Geometry check sheet. Reference: the model listing, model coordinates, mm. A direction names the side the tool comes from. Round coordinates to 2 decimals unless told otherwise and drop trailing zeros. Order: outer loops, then holes, each group sorted by start corner. A loop starts at its lowest first (then second) coordinate and runs counter-clockwise, first axis right, second up.
(1) Cross-section at C-C on z = -2.5. Count the separate pieces of the cut face and the enclosed holes in it, and give its area (3 significant figures).
(2) Gauge pin test, flat ends, axial feed: P1, Ø3.5, axis at x = 0, z = -30.245, coming from the +Y side (3 decimals); P2, Ø3.5, axis at x = 0, y = 22.54, coming from the +Z side; P3, Ø4.5, axis at y = 12, z = -38.5, coming from the +X side. Record the tip position at first contact, or that the pin passes through.
(3) Draft check along Z on faces 6 (the face through (8.372, 1.61, -22.777)), 7 (the face through (0.564, 1.61, -14.112)), 8 (the face through (0, 0, -16)), 9 (the face through (1.3, 20.6, 0)). Enter one of: pulls with the +Z half, pulls with the -Z half, needs draft (parallel to the pull), parting line crosses it, or undercut.
(4) Thickness scan on L1, parallel to Y at x = 0, z = -39.2 (1 decimal); L2, parallel to Y at x = 0, z = -1.9 (1 decimal); L3, parallel to Z at x = 0, y = 1.3 (3 decimals). Record the ranges inside material, lowest first.
(5) Set-up check for faces 1 (the face through (6.35, 14, -38)), 2 (the face through (0.879, 20.852, -1.565)), 3 (the face through (-6.35, 13, -3)), 4 (the face through (-6.35, 13, -38)), 5 (the face through (3, 22, -3.175)): record each of +Z, -Z, +X, -X, +Y, -Y from which the full face is reachable in a straight line by a thin tool's end or side.
(6) Cross-section at B-B on x = -8. Enter the section's corners in (y, z) (3 decimals).
(7) Cross-section at A-A on y = 4.5. Enter the section's corners in (x, z) (3 decimals), and give its area (3 significant figures).
Autodesk Inventor part; units mm, degrees
ref_plane "YZ Plane" through (0, 0, 0) normal (1, 0, 0) x (0, 1, 0)
ref_plane "XZ Plane" through (0, 0, 0) normal (0, 1, 0) x (-1, 0, 0)
ref_plane "XY Plane" through (0, 0, 0) normal (0, 0, 1) x (1, 0, 0)
sketch "Sketch1" plane through (0, 0, 0) normal (0, 0, 1) x (1, 0, 0)
  line L0 (-6.35, 0) -> (-6.35, 3.175)
  line L1 (-6.35, 3.175) -> (-6.35, 34.29)
  line L2 (6.35, 34.29) -> (6.35, 3.175)
  line L3 (6.35, 3.175) -> (6.35, 0)
  line L4 (6.35, 0) -> (-6.35, 0)
  arc A0 (6.35, 34.29) -> (-6.35, 34.29) centre (0, 34.29) ccw
  point P0 (0, 0)
  point P1 (0, 0)
  dimension "d3" = 12.7
  dimension "d4" = 40.64
  dimension "d26" = 6.35
  dimension "d27" = 3.175
extrude "Extrusion1" add sketch "Sketch1" against normal blind 3.175
sketch "Sketch2" plane through (0, 0, -3.175) normal (0, 0, -1) x (-1, 0, 0)
  line L0 (-6.35, 34.29) -> (-6.35, 0)
  line L1 (6.35, 0) -> (-6.35, 0)
  line L2 (-6.35, 0) -> (-6.35, 3.175)
  line L3 (-6.35, 3.175) -> (6.35, 3.175)
  line L4 (6.35, 3.175) -> (6.35, 0)
  point P0 (0, 0)
  point P1 (-6.35, 3.175)
  dimension "d5" = 3.175
extrude "Extrusion2" add sketch "Sketch2" along normal blind 34.452
sketch "Sketch3" plane through (0, 0, -37.627) normal (0, 0, -1) x (-1, 0, 0)
  line L0 (-6.35, 0) -> (6.35, 0)
  line L1 (6.35, 0) -> (-6.35, 0)
  line L2 (6.35, 0) -> (6.35, 34.29)
  line L3 (-6.35, 3.175) -> (-6.35, 0)
  line L4 (-6.35, 0) -> (-6.35, 3.175)
  line L5 (-6.35, 3.175) -> (-6.35, 34.29)
  arc A0 (6.35, 34.29) -> (-6.35, 34.29) centre (0, 34.29) ccw
  point P0 (0, 0)
  dimension "d45" = 6.35
  dimension "d55" = 34.29
extrude "Extrusion7" add sketch "Sketch3" along normal blind 3.175
sketch "Sketch4" plane through (-6.35, 3.175, -3.175) normal (0, 1, 0) x (1, 0, 0)
  circle A0 centre (6.35, 17.226) radius 12.7
  line L0 (0, 0) -> (0, 34.452) construction
  line L1 (0, 0) -> (12.7, 34.452) construction
  point P0 (6.35, -3.175)
  point P1 (12.7, 34.452)
  dimension "d13" = 25.4
extrude "Extrusion4" add sketch "Sketch4" against normal up to surface (3.175 mm away)
sketch "Sketch6" plane through (0, 0, 0) normal (0, 0, 1) x (1, 0, 0)
  circle A0 centre (0, 34.29) radius 1.27
  circle A1 centre (0, 10.795) radius 1.27
  line L0 (0, 10.795) -> (0, 34.29) construction
  line L1 (6.35, 0) -> (-6.35, 0) construction
  line L2 (-1.27, 22.5425) -> (0, 22.5425) construction
  line L3 (-1.27, 10.795) -> (-1.27, 34.29) construction
  arc A2 (6.35, 34.29) -> (-6.35, 34.29) centre (0, 34.29) ccw
  line L4 (-6.35, 3.175) -> (-6.35, 34.29) construction
  line L5 (-6.35, 10.795) -> (6.35, 10.795) construction
  point P0 (0, 0)
  point P1 (0, 0)
  dimension "d18" = 2.54
  dimension "d19" = 23.495
extrude "Extrusion6" cut sketch "Sketch6" against normal blind 500
sketch "Sketch8" plane through (-6.35, 3.175, -3.175) normal (0, 1, 0) x (1, 0, 0)
  circle A0 centre (6.35, 17.226) radius 3.175
  arc A1 (0, 28.2245) -> (0, 6.2275) centre (6.35, 17.226) ccw
  point P0 (6.35, -3.175)
  dimension "d36" = 6.35
extrude "Extrusion9" cut sketch "Sketch8" against normal up to next
sketch "Sketch9" plane through (0, 0, 0) normal (0, 0, 1) x (1, 0, 0)
  circle A0 centre (0, 22.5425) radius 1.905
  circle A1 centre (0, 34.29) radius 1.27 construction
  circle A2 centre (0, 10.795) radius 1.27 construction
  line L0 (0, 34.29) -> (0, 10.795) construction
  point P0 (0, 0)
  point P1 (0, 22.5425)
  dimension "d39" = 3.81
extrude "Extrusion10" cut sketch "Sketch9" against normal up to next
sketch "Sketch10" plane through (-6.35, 3.175, -3.175) normal (0, 1, 0) x (1, 0, 0)
  circle A0 centre (6.35, 10.0521) radius 1.05
  circle A1 centre (-2.159, 18.5611) radius 1.05
  circle A2 centre (6.35, 27.07) radius 1.05
  circle A3 centre (14.859, 18.5611) radius 1.05
  point P0 (6.35, -3.175)
extrude "Extrusion11" cut sketch "Sketch10" against normal up to next
sketch "Sketch12" plane through (0, 0, -40.802) normal (0, 0, -1) x (-1, 0, 0)
  circle A0 centre (0, 22.5425) radius 1.651
  circle A1 centre (0, 22.5425) radius 1.905
  point P0 (0, 0)
  dimension "d52" = 3.302
extrude "Extrusion13" cut sketch "Sketch12" against normal up to next contours A0
properties part number "camerabracket" material "ABS Plastic"
Found:
1. separate pieces: 1
1. enclosed holes: 3
1. area: 477 mm2
2. P1: stops at y = 3.175
2. P2: stops at z = -37.63
2. P3: stops at x = 6.35
3. face 6: undercut
3. face 7: undercut
3. face 8: needs draft
3. face 9: pulls with the +Z half
4. L1: y = 0 to 9.5, 12.1 to 20.9, 24.2 to 33, 35.6 to 40.6
4. L2: y = 0 to 9.5, 12.1 to 20.6, 24.4 to 33, 35.6 to 40.6
4. L3: z = -40.802 to -31.295, -29.195 to -23.576, -17.226 to -14.277, -12.177 to 0
5. face 1: -Z, +X, +Y, -Y
5. face 2: +Z
5. face 3: +Z, -X, +Y, -Y
5. face 4: -Z, -X, +Y, -Y
5. face 5: +X, -X, +Y
6. outline: (0, -30.265) - (3.175, -30.265) - (3.175, -22.654) - (0, -22.654) - close; (0, -20.818) - (3.175, -20.818) - (3.175, -10.537) - (0, -10.537) - close
7. outline: (-6.35, -40.802) - (6.35, -40.802) - (6.35, -37.627) - (-6.35, -37.627) - close; (-6.35, -3.175) - (6.35, -3.175) - (6.35, 0) - (-6.35, 0) - close
7. area: 80.6 mm2
